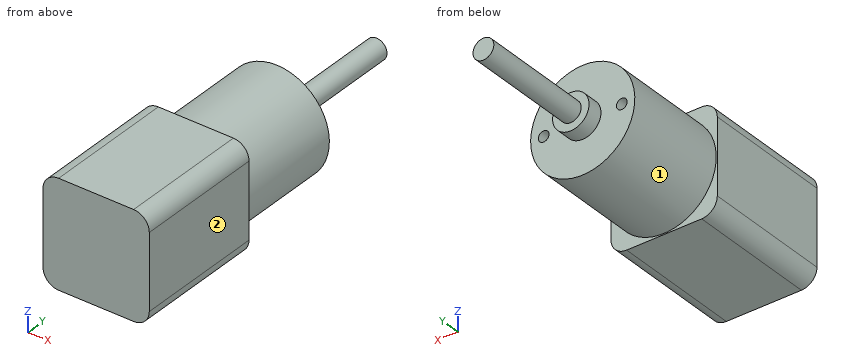
```python
from build123d import *

# Parameters (mm, degrees)
SKETCH2_W               = 20.4
SKETCH2_H               = 20.4
BOSS_EXTRUDE1_DEPTH     = 25.1
SKETCH3_R               = 10
BOSS_EXTRUDE2_DEPTH     = 20.5
SKETCH4_R               = 3.5
BOSS_EXTRUDE3_DEPTH     = 3
SKETCH5_R               = 2
BOSS_EXTRUDE4_DEPTH     = 22
M2_5_TAPPED_HOLE1_D     = 2.05
M2_5_TAPPED_HOLE1_DEPTH = 5
M2_5_TAPPED_HOLE1_TIP   = 0.615882135
FILLET1_R               = 3


with BuildPart() as part:
    # Sketch2 → Boss-Extrude1 (new body)
    with BuildSketch(Plane(origin=(0, 0, 0), x_dir=(1, 0, 0), z_dir=(0, 1, 0))):
        Rectangle(SKETCH2_W, SKETCH2_H)
    extrude(amount=BOSS_EXTRUDE1_DEPTH)

    # Sketch3 → Boss-Extrude2 (add)
    with BuildSketch(Plane(origin=(0, 25.1, 0), x_dir=(1, 0, 0), z_dir=(0, 1, 0))):
        with Locations(Location((0, 0, 0), (0, 0, 270))):
            Circle(SKETCH3_R)
    extrude(amount=BOSS_EXTRUDE2_DEPTH)

    # Sketch4 → Boss-Extrude3 (add)
    with BuildSketch(Plane(origin=(0, 45.6, 0), x_dir=(1, 0, 0), z_dir=(0, 1, 0))):
        with Locations(Location((0, 0, 0), (0, 0, 270))):
            Circle(SKETCH4_R)
    extrude(amount=BOSS_EXTRUDE3_DEPTH)

    # Sketch5 → Boss-Extrude4 (add)
    with BuildSketch(Plane(origin=(0, 48.6, 0), x_dir=(1, 0, 0), z_dir=(0, 1, 0))):
        with Locations(Location((0, 0, 0), (0, 0, 270))):
            Circle(SKETCH5_R)
    extrude(amount=BOSS_EXTRUDE4_DEPTH)

    # M2.5 Tapped Hole1
    with Locations(Plane(origin=(0, 45.6, 0), x_dir=(1, 0, 0), z_dir=(0, 1, 0))):
        with Locations((-7.5, 0), (7.5, 0)):
            Hole(M2_5_TAPPED_HOLE1_D / 2, depth=M2_5_TAPPED_HOLE1_DEPTH)
            with Locations((0, 0, -(M2_5_TAPPED_HOLE1_DEPTH + M2_5_TAPPED_HOLE1_TIP / 2))):  # 118° drill point
                Cone(0, M2_5_TAPPED_HOLE1_D / 2, M2_5_TAPPED_HOLE1_TIP, mode=Mode.SUBTRACT)

    # Fillet1
    fillet1_edges = [part.edges().sort_by_distance(p)[0] for p in [
        (10.2, 12.55, 10.2),
        (-10.2, 12.55, 10.2),
        (-10.2, 12.55, -10.2),
        (10.2, 12.55, -10.2),
    ]]
    fillet(fillet1_edges, radius=FILLET1_R)


solid = part.part
```
The model under review builds one solid part; all positions refer to its coordinate system, in mm. Face numbers are marked on the shaded views. A direction names the side the tool comes from. Round coordinates to 2 decimals unless told otherwise and drop trailing zeros. Order: outer loops, then holes, each group sorted by start corner. A loop starts at its lowest first (then second) coordinate and runs counter-clockwise, first axis right, second up. Notation, with made-up numbers: (21, 62.5) -> (67, 62.5) arc R23 ccw to (67, 92.5) -> close; hole circle Ø1 at (63, 13). An arc over 180 degrees is marked (long way). One line per item, written item: value. Start each with the question number.
Q1. Clearance check with flat-ended pins moving along their axes: pin 1 Ø1.5 at (x, z) = (3, -1) entering from +Y; pin 2 Ø4 at (y, z) = (38, -2) entering from +X; pin 3 Ø10 at (y, z) = (50, 1.5) entering from -X. State where each tip first meets the part, or that it passes through.
Q2. Take a section at B-B (x = 0). Write out the cut boundary in (y, z).
Q3. Take a section at D-D (y = 34). Write out the cut boundary in (x, z).
Q4. Wall thickness on line 1 (Y direction, x = 6.25, z = 6.25); line 2 (Y direction, x = 8, z = -9.5); line 3 (Z direction, x = 7.5, y = 42.8) (3 decimals): over which ranges is each line inside the solid? List them lowest first.
Q5. Take a section at A-A (y = 8.5). Write out the cut boundary in (x, z).
Q6. Take a section at C-C (z = 5.25). Write out the cut boundary in (x, y), and give its area (3 significant figures).
Q7. Machinability: for the marked faces 1 and 2, which of the approach directions +Z, -Z, +X, -X, +Y, -Y give a long, thin tool a straight path to every point of the face, cutting with its end or side? Answer none if there is none.
Reported:
1. pin 1: stops at y = 48.6
1. pin 2: stops at x = 10
1. pin 3: stops at x = -10
2. outline: (0, -10.2) -> (25.1, -10.2) -> (25.1, -10) -> (45.6, -10) -> (45.6, -3.5) -> (48.6, -3.5) -> (48.6, -2) -> (70.6, -2) -> (70.6, 2) -> (48.6, 2) -> (48.6, 3.5) -> (45.6, 3.5) -> (45.6, 10) -> (25.1, 10) -> (25.1, 10.2) -> (0, 10.2) -> close
3. outline: circle Ø20 at (0, 0)
4. line 1: y = 0 to 45.6
4. line 2: y = 0 to 25.1
4. line 3: z = -6.614 to -1.025, 1.025 to 6.614
5. outline: (-10.2, -7.2) arc R3 ccw to (-7.2, -10.2) -> (7.2, -10.2) arc R3 ccw to (10.2, -7.2) -> (10.2, 7.2) arc R3 ccw to (7.2, 10.2) -> (-7.2, 10.2) arc R3 ccw to (-10.2, 7.2) -> close
6. outline: (-10.2, 0) -> (10.2, 0) -> (10.2, 25.1) -> (8.51, 25.1) -> (8.51, 45.6) -> (-8.51, 45.6) -> (-8.51, 25.1) -> (-10.2, 25.1) -> close
6. area: 861 mm2
7. face 1: +Y
7. face 2: +Z, -Z, +X, +Y, -Y
